Autodesk Inventor part; units mm, degrees
ref_plane "YZ Plane" through (0, 0, 0) normal (1, 0, 0) x (0, 1, 0)
ref_plane "XZ Plane" through (0, 0, 0) normal (0, 1, 0) x (-1, 0, 0)
ref_plane "XY Plane" through (0, 0, 0) normal (0, 0, 1) x (1, 0, 0)
sketch "Sketch1" plane through (0, 0, 0) normal (0, 0, 1) x (1, 0, 0)
  line L0 (0, 0) -> (0, 45)
  line L1 (19, 0) -> (19, 45)
  line L2 (19, 45) -> (25, 45)
  line L3 (25, 45) -> (25, 34.25)
  line L4 (25, 34.25) -> (40, 34.25)
  line L5 (40, 24.25) -> (25, 24.25)
  line L6 (25, 24.25) -> (25, 0)
  line L7 (25, 0) -> (19, 0)
  arc A0 (40, 24.25) -> (40, 34.25) centre (40, 29.25) ccw
  point P0 (45, 29.25)
  dimension "d2" = 45
  dimension "d3" = 38
  dimension "d4" = 6
  dimension "d6" = 10
  dimension "d8" = 90
revolve "Revolution1" add sketch "Sketch1" angle 360 about axis through (0, 0, 0) along (0, 1, 0)
fillet "Fillet1" radius 5 2 edges at (-25, 34.25, 0) (-25, 24.25, 0)
thread "Thread1"
properties part number "nut" material "Brass, Soft Yellow, Welded"
Part model, mm, in its own coordinate system. A direction names the side the tool comes from. Coordinates: 2 decimals unless noted, no trailing zeros. Write each loop counter-clockwise with the first axis right and the second up, starting at its lowest first coordinate (ties: lowest second). Pieces come first, ordered by that corner, then holes.
Item 1: Slice it at B-B (x = 0). Write the cut outline in (y, z).
Item 2: Probe line 1 (Y direction, x = 30, z = 17); line 2 (Y direction, x = -20, z = -35); line 3 (X direction, y = 16, z = 0). List the from-to ranges inside material, lowest first.
Item 3: Mould opens along Z. For faces 4 (the face through (8.767, 22.815, 16.856)), 5 (the face through (23.846, 9.49, 7.509)), 6 (the face through (-4, 0, -19)) say: released by +Z, released by -Z, zero draft, split by the parting line, or undercut.
Item 4: Slice it at C-C (y = 10). Write the cut outline in (x, z).
Item 5: Slice it at A-A (z = 0). Write the cut outline in (x, y).
Item 6: Pin check, flat tips, straight feed: pin 1 (10 mm diameter, centred on x = 8.5, y = 38, fed in from -Z); pin 2 (12 mm diameter, centred on y = 6, z = -6, fed in from -X); pin 3 (5 mm diameter, centred on y = 12, z = 16.5, fed in from -X). Stop position of each tip, or through.
Item 7: Which spindle directions (+Z, -Z, +X, -X, +Y, -Y) get a long thin tool onto all of the face, cutting with end or side? Do faces 1 (the face through (6, 34.25, -30)), 2 (the face through (-4, 45, -19)), 3 (the face through (6, 24.25, -30)). Say none if no direction does.
Results found:
1. outline: (0, -25) - (19.25, -25) arc R5 cw to (24.25, -30) - (24.25, -40) arc R5 ccw to (34.25, -40) - (34.25, -30) arc R5 cw to (39.25, -25) - (45, -25) - (45, -19) - (0, -19) - close; (0, 19) - (45, 19) - (45, 25) - (39.25, 25) arc R5 cw to (34.25, 30) - (34.25, 40) arc R5 ccw to (24.25, 40) - (24.25, 30) arc R5 cw to (19.25, 25) - (0, 25) - close
2. line 1: y = 24.25 to 34.25
2. line 2: y = 24.26 to 34.24
2. line 3: x = -25 to -19, 19 to 25
3. face 4: undercut
3. face 5: split by the parting line
3. face 6: zero draft
4. outline: circle Ø50 at (0, 0); hole circle Ø38 at (0, 0)
5. outline: (-40, 24.25) - (-30, 24.25) arc R5 cw to (-25, 19.25) - (-25, 0) - (-19, 0) - (-19, 45) - (-25, 45) - (-25, 39.25) arc R5 cw to (-30, 34.25) - (-40, 34.25) arc R5 ccw to start; (19, 0) - (25, 0) - (25, 19.25) arc R5 cw to (30, 24.25) - (40, 24.25) arc R5 ccw to (40, 34.25) - (30, 34.25) arc R5 cw to (25, 39.25) - (25, 45) - (19, 45) - close
6. pin 1: stops at z = -42.54
6. pin 2: stops at x = -25
6. pin 3: stops at x = -20.71
7. face 1: +Y
7. face 2: +Z, -Z, +X, -X, +Y
7. face 3: -Y
